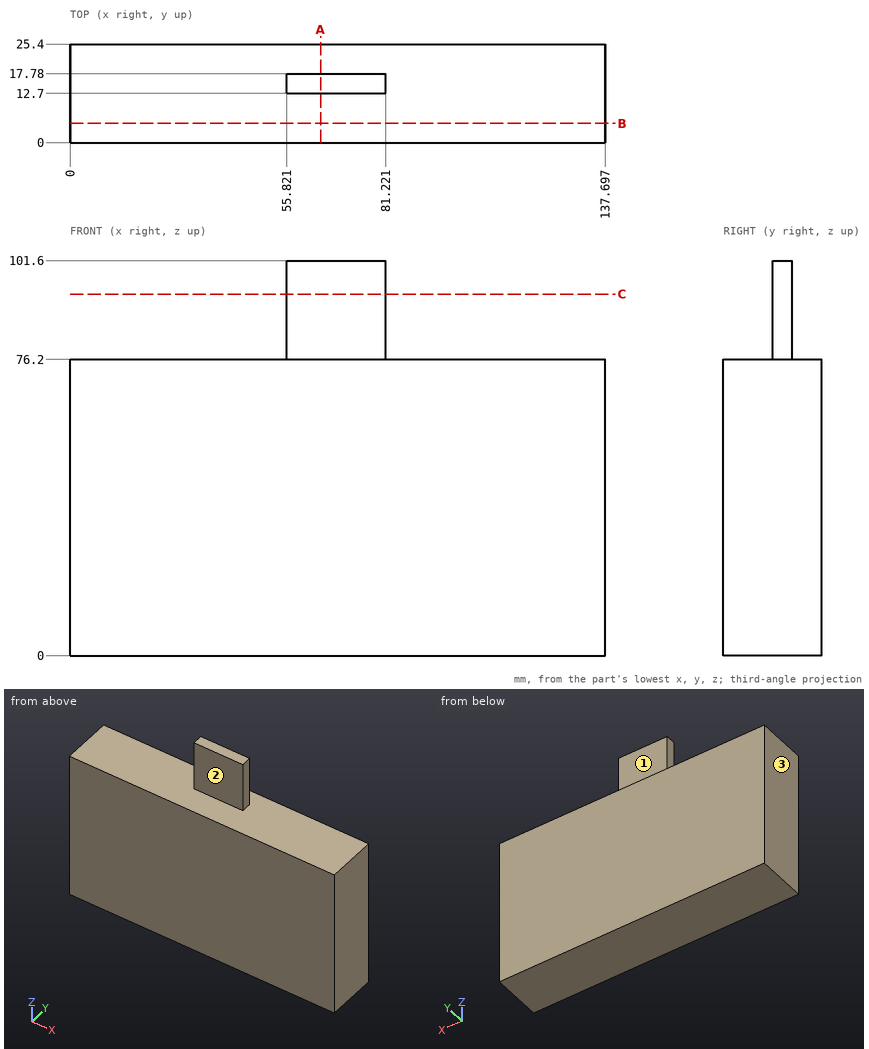
Study the drawing (mm; zero at the part's minimum x, y, z) and answer. A direction names the side the tool comes from. Give positions to 0.01 mm unless a question says otherwise; leave off trailing zeros. Write each loop counter-clockwise with the first axis right and the second up, starting at its lowest first coordinate (ties: lowest second). Pieces come first, ordered by that corner, then holes.
(1) The part is cut by section B-B on y = 5. Write down the section's boundary in (x, z), plus the area to 3 significant figures.
Final values:
outline: (0, 0) - (137.7, 0) - (137.7, 76.2) - (0, 76.2) - close
area: 10,500 mm2
(2) The part is cut by section C-C on z = 93. Write down the section's boundary in (x, y).
Final values:
outline: (55.82, 12.7) - (81.22, 12.7) - (81.22, 17.78) - (55.82, 17.78) - close
(3) The part is cut by section A-A on x = 64.5. Write down the section's boundary in (y, z), plus the area to 3 significant figures.
Final values:
outline: (0, 0) - (25.4, 0) - (25.4, 76.2) - (17.78, 76.2) - (17.78, 101.6) - (12.7, 101.6) - (12.7, 76.2) - (0, 76.2) - close
area: 2,060 mm2
(4) Flat-ended cylindrical pins translate along their axes: pin 1 Ø5 at (x, y) = (16, 4.5) entering from +Z; pin 2 Ø12 at (x, z) = (83.5, 89) entering from +Y; pin 3 Ø1.5 at (y, z) = (15.5, 90.5) entering from -X. Find the tip coordinate at first contact, or state that the pin passes through.
Final values:
pin 1: stops at z = 76.2
pin 2: stops at y = 17.78
pin 3: stops at x = 55.82
(5) Which of the six approach directions +Z, -Z, +X, -X, +Y, -Y give full straight-line access (tool end or side, diameter ignored) to the marked faces 1, 2 and 3?
Final values:
face 1: +Z, +X, -X, +Y
face 2: +Z, +X, -X, -Y
face 3: +Z, -Z, -X, +Y, -Y
(6) Straight lines are drawn through the part: line 1 (Z direction, x = 121, y = 1.5); line 2 (X direction, y = 17.5, z = 87). For each, find the intervals that lie inside material, in ascending order.
Final values:
line 1: z = 0 to 76.2
line 2: x = 55.82 to 81.22
